Autodesk Fusion 360 part; units mm, degrees
sketch "Sketch1" plane through (0, 0, 0) normal (0, 0, 1) x (1, 0, 0)
  line L0 (0, 0) -> (100, 0)
  line L1 (100, 0) -> (100, 50)
  line L2 (100, 50) -> (0, 50)
  line L3 (0, 50) -> (0, 0)
  line L4 (0, 0) -> (100, 0)
  line L5 (100, 0) -> (100, 18.5)
  line L6 (100, 18.5) -> (0, 18.5)
  line L7 (0, 18.5) -> (0, 0)
  line L8 (0, 50) -> (100, 50)
  line L9 (100, 50) -> (100, 31.5)
  line L10 (100, 31.5) -> (0, 31.5)
  line L11 (0, 31.5) -> (0, 50)
  dimension "d1" = 100
  dimension "d2" = 50
  dimension "d3" = 18.5
  dimension "d4" = 18.5
extrude "Extrude1" add sketch "Sketch1" along normal blind 3 contours L1 L3 L6 L10
extrude "Extrude2" add sketch "Sketch1" along normal blind 40 contours L0 L1 L3 L4 L5 L6 L7 | L1 L2 L3 L8 L9 L10 L11
sketch "Sketch2" plane through (100, 0, 0) normal (1, 0, 0) x (0, 1, 0)
  line L0 (0, 0) -> (50, 0)
  line L1 (50, 0) -> (50, 40)
  line L2 (50, 40) -> (31.5, 40)
  line L3 (31.5, 40) -> (31.5, 3)
  line L4 (31.5, 3) -> (18.5, 3)
  line L5 (18.5, 3) -> (18.5, 40)
  line L6 (18.5, 40) -> (0, 40)
  line L7 (0, 40) -> (0, 0)
  line L8 (18.5, 40) -> (15.5, 40)
  line L9 (31.5, 40) -> (34.5, 40)
  spline S0 degree 5 poles (0, 3) (0.6686, 2.9687) (1.9704, 2.982) (3.8176, 3.2291) (6.0657, 4.0208) (8.4986, 5.8217) (10.5348, 8.4758) (12.1729, 11.9864) (13.442, 16.2906) (14.3808, 21.3051) (15.0282, 26.9468) (15.3373, 31.909) (15.4603, 35.8649) (15.4947, 38.6046) (15.5, 40) knots 0 0 0 0 0 0 0.1 0.2 0.3 0.4 0.5 0.6 0.7 0.8 0.9 1 1 1 1 1 1
  spline S1 degree 5 poles (50, 3) (49.3314, 2.9687) (48.0296, 2.982) (46.1824, 3.2291) (43.9343, 4.0208) (41.5014, 5.8217) (39.4652, 8.4758) (37.8271, 11.9864) (36.558, 16.2906) (35.6192, 21.3051) (34.9718, 26.9468) (34.6627, 31.909) (34.5397, 35.8649) (34.5053, 38.6046) (34.5, 40) knots 0 0 0 0 0 0 0.1 0.2 0.3 0.4 0.5 0.6 0.7 0.8 0.9 1 1 1 1 1 1
  line L10 (34.5, 40) -> (50, 40)
  line L11 (50, 3) -> (50, 40)
  line L12 (0, 3) -> (0, 40)
  line L13 (15.5, 40) -> (0, 40)
  point P0 (10, 8)
  point P1 (40, 8)
  dimension "d9" = 3
  dimension "d10" = 3
extrude "Extrude3" cut sketch "Sketch2" against normal blind 100 contours L6 L7 S0 L12 L13 | L1 L2 S1 L10 L11
Read the model definition and answer for the solid it produces. Units are mm, in the model's axes. A direction names the side the tool comes from. Coordinates: 2 decimals unless noted, no trailing zeros. Loops run counter-clockwise (first coordinate to the right, second up) from the corner with the lowest first, then second, coordinate; pieces in that order, holes last. Notation, with made-up numbers: (8.5, 70) -> (18.5, 70) arc R32 cw to (18.5, 102) -> close; hole circle Ø7 at (58.25, 66.25). An arc over 180 degrees is marked (long way). Return JSON: item names as keys, results as strings.
Item 1: Find section A-A (y = 27). Determine the outline of the cut face in (x, z), plus the area to 3 significant figures.
Answers:
{"outline": "(0, 0) -> (100, 0) -> (100, 3) -> (0, 3) -> close", "area": "300 mm2"}
Item 2: For faces 4 (the flat face through (100, 32, 11)), 5 (the flat face through (49, 25, 3)), determine the directions among +Z, -Z, +X, -X, +Y, -Y from which every point of the face is accessible in a straight line to the end or side of a thin tool.
Answers:
{"face 4": "+Z, -Z, +X, +Y, -Y", "face 5": "+Z, +X, -X"}
Item 3: Flat-ended cylindrical pins translate along their axes: P1, Ø18.5, axis at x = 33.5, z = 29.5, coming from the -Y side; P2, Ø3, axis at x = 58, y = 26.5, coming from the +Z side; P3, Ø1, axis at x = 10.5, z = 27.5, coming from the +Y side; P4, Ø12, axis at x = 88.5, y = 15, coming from the -Z side. Find the tip coordinate at first contact, or state that the pin passes through.
Answers:
{"P1": "stops at y = 14.12", "P2": "stops at z = 3", "P3": "stops at y = 35.04", "P4": "stops at z = 0"}
Item 4: Find the intervals of material crossed by probe 1 along Z at (x, y) = (11, 24.5); probe 2 along Y at (x, z) = (66.5, 17); probe 3 along Y at (x, z) = (21, 7), in increasing order.
Answers:
{"probe 1": "z = 0 to 3", "probe 2": "y = 13.48 to 18.5, 31.5 to 36.52", "probe 3": "y = 9.27 to 18.5, 31.5 to 40.73"}
Item 5: For a pull along Y with two mould halves and no side action, classify faces 1 (the flat face through (51, 31.5, 21)), 2 (the flat face through (51, 50, 1)), 3 (the flat face through (49, 17, 40)) as +Y half, -Y half, draft (parallel to the pull), parting line (faces both ways), or undercut.
Answers:
{"face 1": "undercut", "face 2": "+Y half", "face 3": "draft"}
